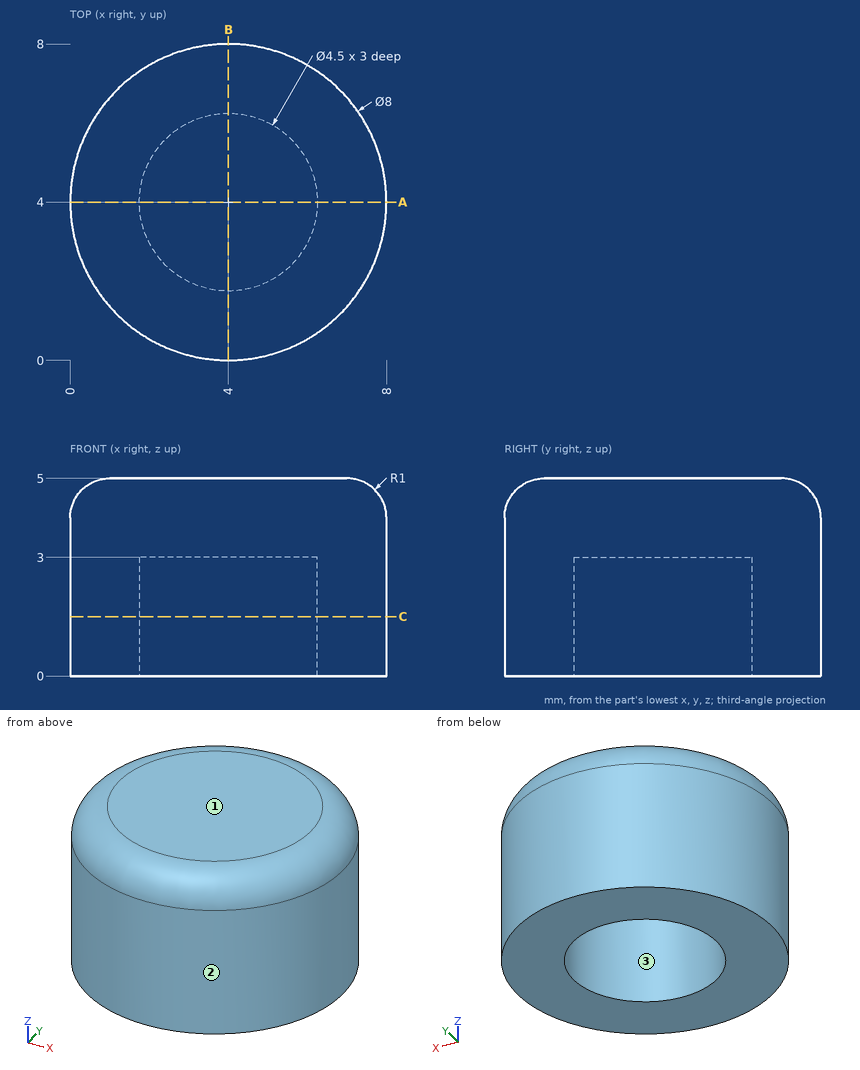
Geometry check sheet. Reference: drawing and pictorial views, mm from the part's lowest x, y, z. Coordinates: 2 decimals unless noted, no trailing zeros. Write each loop counter-clockwise with the first axis right and the second up, starting at its lowest first coordinate (ties: lowest second). Pieces come first, ordered by that corner, then holes. Notation, with made-up numbers: M 72.5,-13.75 L 97.5,-13.75 A22 ccw 97.5,-3.75 Z; hole C 77.25,53 d10. An arc over 180 degrees is marked long. Use one line per item in the form item = value.
Item 1: Material ranges on L1, parallel to Y at x = 4, z = 1.8; L2, parallel to Z at x = 4, y = 6; L3, parallel to X at y = 5.5, z = 0.85, recorded low to high. Write a range as from..to.
Answer below:
L1 = 0..1.75, 6.25..8
L2 = 3..5
L3 = 0.29..2.32, 5.68..7.71
Item 2: Sectioned sample at A-A, the plane y = 4. Record the cut outline in (x, z), and give its area (3 significant figures).
Answer below:
outline = M 0,0 L 1.75,0 L 1.75,3 L 6.25,3 L 6.25,0 L 8,0 L 8,4 A1 ccw 7,5 L 1,5 A1 ccw 0,4 Z
area = 26.1 mm^2
Item 3: Gauge pin test, flat ends, axial feed: pin 1 Ø3 at (x, y) = (2, 1.5) entering from +Z; pin 2 Ø3.5 at (x, y) = (4, 4) entering from -Z. Record the tip position at first contact, or that the pin passes through.
Answer below:
pin_1 = 5
pin_2 = 3
Item 4: Sectioned sample at C-C, the plane z = 1.5. Record the cut outline in (x, y).
Answer below:
outline = C 4,4 d8; hole C 4,4 d4.5
Item 5: Release check for a two-part mould opening along Y. For the marked faces 1, 2 and 3 record: pulls with the +Y half, pulls with the -Y half, needs draft (parallel to the pull), parting line crosses it, or undercut.
Answer below:
face_1 = needs draft
face_2 = parting line crosses it
face_3 = undercut
